```python
from build123d import *

# Parameters (mm, degrees)
CROQUIS1_R              = 5
SALIENTE_EXTRUIR1_DEPTH = 10
ESCALA1_SCALE           = 0.75


with BuildPart() as part:
    # Croquis1 → Saliente-Extruir1 (new body)
    with BuildSketch(Plane(origin=(0, 0, 0), x_dir=(1, 0, 0), z_dir=(0, 1, 0))):
        with BuildLine():
            Line((0, 7.5), (30, 7.5))
            ThreePointArc((30, 7.5), (37.5, 0), (30, -7.5))
            Line((30, -7.5), (0, -7.5))
            ThreePointArc((0, -7.5), (-7.5, 0), (0, 7.5))
        make_face()
        with Locations(Location((0, 0, 0), (0, 0, 270))):
            Circle(CROQUIS1_R, mode=Mode.SUBTRACT)
        with Locations(Location((30, 0, 0), (0, 0, 270))):
            Circle(CROQUIS1_R, mode=Mode.SUBTRACT)
    extrude(amount=SALIENTE_EXTRUIR1_DEPTH)


with BuildPart() as part_1:
    # Escala1: scaled about (15, 5, 0)
    add(part.part.scale(ESCALA1_SCALE).moved(Location((3.75, 1.25, 0))))


solid = part_1.part
```
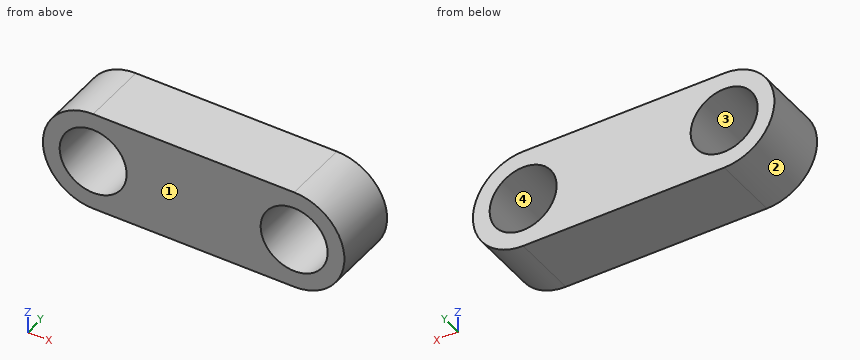
Design review of the part built by this model. Coordinates are the model's own, in mm. Face numbers are marked on the shaded views. Give positions to 0.01 mm unless a question says otherwise; leave off trailing zeros. Order: outer loops, then holes, each group sorted by start corner. A loop starts at its lowest first (then second) coordinate and runs counter-clockwise, first axis right, second up. Notation, with made-up numbers: (65.25, 21) -> (104.25, 21) arc R25 ccw to (104.25, 41) -> close; hole circle Ø2 at (40.25, 3.25). An arc over 180 degrees is marked (long way). Write item = value, one per line. Start each with the question number.
(1) We need section D-D on z = 0. Write out the cut boundary in (x, y) (3 decimals), plus the area to 3 significant figures.
(2) For pin 1 (1 mm diameter, centred on x = 28, y = 4, fed in from -Z); pin 2 (2 mm diameter, centred on y = 2, z = 4, fed in from +X), all flat-tipped, find the tip position at first contact; note any pin that passes through.
(3) We need section C-C on y = 4.5. Write out the cut boundary in (x, z) (3 decimals), plus the area to 3 significant figures.
(4) We need section B-B on x = 3. Write out the cut boundary in (y, z), plus the area to 3 significant figures.
(5) To check wall thickness, follow line 1 along X through (y, z) = (5.75, 0) (3 decimals); line 2 along X through (y, z) = (3.5, 1.5); line 3 along Z through (x, y) = (25.5, 5.5) (3 decimals). State the ranges of each line that lie inside material, in increasing order.
(6) We need section A-A on z = 3.25. Write out the cut boundary in (x, y), plus the area to 3 significant figures.
(7) Mouldability with a two-part tool opening along X and no side actions: class the marked faces 1, 2, 3 and 4 as +X half, -X half, draft (parallel to the pull), parting line (faces both ways), or undercut.
Numbers:
q1.outline = (-1.875, 1.25) -> (0, 1.25) -> (0, 8.75) -> (-1.875, 8.75) -> close; (7.5, 1.25) -> (22.5, 1.25) -> (22.5, 8.75) -> (7.5, 8.75) -> close; (30, 1.25) -> (31.875, 1.25) -> (31.875, 8.75) -> (30, 8.75) -> close
q1.area = 141 mm^2
q2.pin_1 = -5.48
q2.pin_2 = 31.01
q3.outline = (3.75, -5.625) -> (26.25, -5.625) arc R5.625 ccw to (26.25, 5.625) -> (3.75, 5.625) arc R5.625 ccw to start; hole circle Ø7.5 at (3.75, 0); hole circle Ø7.5 at (26.25, 0)
q3.area = 264 mm^2
q4.outline = (1.25, -5.57) -> (8.75, -5.57) -> (8.75, -3.67) -> (1.25, -3.67) -> close; (1.25, 3.67) -> (8.75, 3.67) -> (8.75, 5.57) -> (1.25, 5.57) -> close
q4.area = 28.5 mm^2
q5.line_1 = -1.875 to 0, 7.5 to 22.5, 30 to 31.875
q5.line_2 = -1.67 to 0.31, 7.19 to 22.81, 29.69 to 31.67
q5.line_3 = -5.625 to -3.674, 3.674 to 5.625
q6.outline = (-0.84, 1.25) -> (1.88, 1.25) -> (1.88, 8.75) -> (-0.84, 8.75) -> close; (5.62, 1.25) -> (24.38, 1.25) -> (24.38, 8.75) -> (5.62, 8.75) -> close; (28.12, 1.25) -> (30.84, 1.25) -> (30.84, 8.75) -> (28.12, 8.75) -> close
q6.area = 181 mm^2
q7.face_1 = draft
q7.face_2 = -X half
q7.face_3 = undercut
q7.face_4 = undercut
